Autodesk Inventor part; units mm, degrees
ref_plane "YZ Plane" through (0, 0, 0) normal (1, 0, 0) x (0, 1, 0)
ref_plane "XZ Plane" through (0, 0, 0) normal (0, 1, 0) x (-1, 0, 0)
ref_plane "XY Plane" through (0, 0, 0) normal (0, 0, 1) x (1, 0, 0)
sketch "スケッチ1" plane through (0, 0, 0) normal (0, 1, 0) x (-1, 0, 0)
  line L0 (46, 50) -> (-46, 50) construction
  line L1 (-46, 50) -> (-46, -50) construction
  line L2 (-46, -50) -> (46, -50) construction
  line L3 (46, -50) -> (46, 50) construction
  line L4 (46, 50) -> (-46, -50) construction
  line L5 (-46, 50) -> (46, -50) construction
  circle A0 centre (41, -44) radius 1.5
  line L6 (45, 22) -> (-45, 22) construction
  line L7 (-45, 22) -> (-45, -48) construction
  line L8 (-45, -48) -> (45, -48) construction
  line L9 (45, -48) -> (45, 22) construction
  circle A1 centre (41, 18) radius 1.5
  circle A2 centre (-41, 18) radius 1.5
  circle A3 centre (-41, -44) radius 1.5
  line L10 (48, 0) -> (48, -20)
  line L11 (48, -20) -> (46, -20)
  line L12 (46, -20) -> (46, -35)
  line L13 (46, -35) -> (48, -35)
  line L14 (48, -35) -> (48, -52)
  line L15 (0, 0) -> (80.4536, 0) construction
  line L16 (48, 0) -> (48, 20)
  line L17 (48, 20) -> (46, 20)
  line L18 (46, 20) -> (46, 35)
  line L19 (46, 35) -> (48, 35)
  line L20 (48, 35) -> (48, 52)
  line L21 (0, 0) -> (0, 71.6244) construction
  line L22 (-48, 0) -> (-48, -20)
  line L23 (-48, -20) -> (-46, -20)
  line L24 (-46, -20) -> (-46, -35)
  line L25 (-46, -35) -> (-48, -35)
  line L26 (-48, -35) -> (-48, -52)
  line L27 (-48, 0) -> (-48, 20)
  line L28 (-48, 20) -> (-46, 20)
  line L29 (-46, 20) -> (-46, 35)
  line L30 (-46, 35) -> (-48, 35)
  line L31 (-48, 35) -> (-48, 52)
  line L32 (48, 52) -> (31, 52)
  line L33 (31, 52) -> (31, 50)
  line L34 (31, 50) -> (16, 50)
  line L35 (16, 50) -> (16, 52)
  line L36 (16, 52) -> (0, 52)
  line L37 (-48, 52) -> (-31, 52)
  line L38 (-31, 52) -> (-31, 50)
  line L39 (-31, 50) -> (-16, 50)
  line L40 (-16, 50) -> (-16, 52)
  line L41 (-16, 52) -> (0, 52)
  line L42 (46, -50) -> (-46, -50) construction
  line L43 (48, -52) -> (31, -52)
  line L44 (31, -52) -> (31, -50)
  line L45 (31, -50) -> (16, -50)
  line L46 (16, -50) -> (16, -52)
  line L47 (16, -52) -> (0, -52)
  line L48 (-16, -52) -> (0, -52)
  line L49 (-16, -50) -> (-16, -52)
  line L50 (-31, -50) -> (-16, -50)
  line L51 (-31, -52) -> (-31, -50)
  line L52 (-48, -52) -> (-31, -52)
  dimension "d0" = 92
  dimension "d1" = 100
  dimension "d2" = 3
  dimension "d5" = 90
  dimension "d6" = 70
  dimension "d7" = 1
  dimension "d8" = 2
  dimension "d9" = 3
  dimension "d10" = 4
  dimension "d11" = 4
  dimension "d12" = 4
  dimension "d13" = 4
  dimension "d14" = 3
  dimension "d15" = 3
  dimension "d16" = 4
  dimension "d17" = 4
  dimension "d18" = 4
  dimension "d19" = 4
  dimension "d32" = 17
  dimension "d33" = 15
  dimension "d34" = 20
  dimension "d35" = 2
  dimension "d36" = 2
  dimension "d37" = 17
  dimension "d38" = 15
  dimension "d39" = 16
  dimension "d40" = 2
  dimension "d41" = 2
extrude "押し出し1" add sketch "スケッチ1" along normal mid plane 2
equation "\"d9\" = d2"
equation "\"d10\" = d11"
equation "\"d13\" = d12"
equation "\"d14\" = d2"
equation "\"d15\" = d2"
equation "\"d16\" = d11"
equation "\"d17\" = d10"
equation "\"d18\" = d11"
equation "\"d19\" = d10"
equation "\"d36\" = d35"
properties part number "Back"
Geometry check sheet. Reference: the model listing, model coordinates, mm. Give positions to 0.01 mm unless a question says otherwise; leave off trailing zeros. Loops run counter-clockwise (first coordinate to the right, second up) from the corner with the lowest first, then second, coordinate; pieces in that order, holes last. Notation, with made-up numbers: M -35,21 L 15,21 A23 cw 15,57 Z; hole C 20.25,-12 d3. An arc over 180 degrees is marked long. Answer as CSV lines item,"result".
Item 1: Release check for a two-part mould opening along X. For faces 1 (the flat face through (1, -1, 1)), 2 (the cylindrical face through (-39.8, 0, -43.1)) record: pulls with the +X half, pulls with the -X half, needs draft (parallel to the pull), parting line crosses it, or undercut.
Values:
face 1,"needs draft"
face 2,"undercut"
Item 2: Cross-section at C-C on z = 33. Record the cut outline in (x, y), and give its area (3 significant figures).
Values:
outline,"M -46,-1 L 46,-1 L 46,1 L -46,1 Z"
area,"184 mm²"
Item 3: Cross-section at A-A on z = -44. Record the cut outline in (x, y).
Values:
outline,"M -48,-1 L -42.5,-1 L -42.5,1 L -48,1 Z; M -39.5,-1 L 39.5,-1 L 39.5,1 L -39.5,1 Z; M 42.5,-1 L 48,-1 L 48,1 L 42.5,1 Z"
Item 4: Material ranges on line 1 (Z direction, x = -41, y = 0.3); line 2 (Z direction, x = -40.5, y = -0.35); line 3 (Z direction, x = 30, y = -0.7), recorded low to high.
Values:
line 1,"z = -52 to -45.5, -42.5 to 16.5, 19.5 to 52"
line 2,"z = -52 to -45.41, -42.59 to 16.59, 19.41 to 52"
line 3,"z = -50 to 50"
Item 5: Cross-section at D-D on x = 24. Record the cut outline in (y, z), and give its area (3 significant figures).
Values:
outline,"M -1,-50 L 1,-50 L 1,50 L -1,50 Z"
area,"200 mm²"
Item 6: Depth check by flat-ended pin: P1, Ø1, axis at y = 0.5, z = 28.5, coming from the -X side. Enter the tip coordinate at first touch or a pass-through.
Values:
P1,"stops at x = -46"
Item 7: Cross-section at B-B on x = 41. Record the cut outline in (y, z).
Values:
outline,"M -1,-52 L 1,-52 L 1,-45.5 L -1,-45.5 Z; M -1,-42.5 L 1,-42.5 L 1,16.5 L -1,16.5 Z; M -1,19.5 L 1,19.5 L 1,52 L -1,52 Z"
